```python
from build123d import *

# Parameters (mm, degrees)
SKETCH1_W           = 80
SKETCH1_H           = 80
SKETCH1_R           = 20
BOSS_EXTRUDE1_DEPTH = 40
SKETCH1_3_R         = 20
BOSS_EXTRUDE2_DEPTH = 60


with BuildPart() as part:
    # Sketch1 → Boss-Extrude1 (new body)
    with BuildSketch(Plane(origin=(0, 0, 0), x_dir=(1, 0, 0), z_dir=(0, 1, 0))):
        with Locations((40, 40)):
            Rectangle(SKETCH1_W, SKETCH1_H)
        with Locations((40, 40)):
            Circle(SKETCH1_R, mode=Mode.SUBTRACT)
    extrude(amount=BOSS_EXTRUDE1_DEPTH)

    # Sketch1<3> → Boss-Extrude2 (add)
    with BuildSketch(Plane(origin=(0, 0, 0), x_dir=(1, 0, 0), z_dir=(0, 1, 0))):
        with Locations((40, 40)):
            Circle(SKETCH1_3_R)
    extrude(amount=BOSS_EXTRUDE2_DEPTH)


solid = part.part
```
Part model, mm, in its own coordinate system. A direction names the side the tool comes from. Give positions to 0.01 mm unless a question says otherwise; leave off trailing zeros. Write each loop counter-clockwise with the first axis right and the second up, starting at its lowest first coordinate (ties: lowest second). Pieces come first, ordered by that corner, then holes. Notation, with made-up numbers: (-32.5, -3.5) -> (-22.5, -3.5) arc R21 cw to (-22.5, 19.5) -> close; hole circle Ø4 at (15, -34). An arc over 180 degrees is marked (long way). Put each result on its own line as item: value. Start each with the question number.
Item 1: Wall check: L1, parallel to Y at x = 65.5, z = -13.5; L2, parallel to X at y = 53, z = -40; L3, parallel to X at y = 40.5, z = -46. Give the ranges that are in metal, low to high. Write a range as [from, to].
Item 2: Cut at B-B (x = 40). List the corners of the cut face in (y, z).
Item 3: Pin check, flat tip, straight feed: pin 1 Ø3 at (x, y) = (56, 46.5) entering from +Z (3 decimals). Stop position of the tip, or through.
Item 4: Cut at A-A (z = -40). List the corners of the cut face in (x, y).
Item 5: Cut at C-C (z = -9.5). List the corners of the cut face in (x, y).
Item 6: Which spindle directions (+Z, -Z, +X, -X, +Y, -Y) get a long thin tool onto all of the face, cutting with end or side? Do faces 1 (the face through (39, 0, -41)), 2 (the face through (59.076, 49.86, -46.007)). Say none if no direction does.
Answer list:
1. L1: y = [0, 40]
1. L2: x = [20, 60]
1. L3: x = [20.92, 59.08]
2. outline: (0, -80) -> (40, -80) -> (40, -60) -> (60, -60) -> (60, -20) -> (40, -20) -> (40, 0) -> (0, 0) -> close
3. pin 1: stops at z = -26.225
4. outline: (0, 0) -> (80, 0) -> (80, 40) -> (60, 40) -> (60, 60) -> (20, 60) -> (20, 40) -> (0, 40) -> close
5. outline: (0, 0) -> (80, 0) -> (80, 40) -> (0, 40) -> close
6. face 1: +Z, -Z, +X, -X, -Y
6. face 2: +Y
